CAD build for the part. Positions are in the model's coordinates, mm. Face numbers are marked on the shaded views. Coordinates: 2 decimals unless noted, no trailing zeros. Order: outer loops, then holes, each group sorted by start corner. A loop starts at its lowest first (then second) coordinate and runs counter-clockwise, first axis right, second up. Notation, with made-up numbers: (75, 3.25) -> (115, 3.25) arc R8 ccw to (115, 10.25) -> close; hole circle Ø4 at (81.25, 45.5). An arc over 180 degrees is marked (long way). Use one line per item in the form item = value. Start each with the question number.
from build123d import *

# Parameters (mm, degrees)
F1_DEPTH = 60
F2_R     = 26.678258
F3_DEPTH = 25


with BuildPart() as f1:
    # F0 (on Front) → F1 (new body)
    with BuildSketch(Plane.XZ):
        with BuildLine():
            Line((4.061145, 78.143452), (-15.64565, 78.143452))
            ThreePointArc((-15.64565, 78.143452), (-26.968879, 75.432115), (-35.83602, 67.886212))
            Line((-35.83602, 67.886212), (-50.667426, 47.57444))
            ThreePointArc((-50.667426, 47.57444), (-54.244252, 40.585414), (-55.477056, 32.831681))
            Line((-55.477056, 32.831681), (-55.477056, 3.143452))
            ThreePointArc((-55.477056, 3.143452), (-48.154725, -14.534217), (-30.477056, -21.856548))
            Line((-30.477056, -21.856548), (19.522944, -21.856548))
            ThreePointArc((19.522944, -21.856548), (37.200614, -14.534217), (44.522944, 3.143452))
            Line((44.522944, 3.143452), (44.522944, 32.623266))
            ThreePointArc((44.522944, 32.623266), (43.231192, 40.555414), (39.489426, 47.667853))
            Line((39.489426, 47.667853), (24.027628, 68.188039))
            ThreePointArc((24.027628, 68.188039), (15.216533, 75.516591), (4.061145, 78.143452))
        make_face()
    extrude(amount=F1_DEPTH)

    # F2 (on face) → F3 (cut)
    with BuildSketch(Plane(origin=(0, 0, 0), x_dir=(-1, 0, 0), z_dir=(0, 1, 0))):
        with Locations((6.659664, 24.698926)):
            Circle(F2_R)
    extrude(amount=-F3_DEPTH, mode=Mode.SUBTRACT)


solid = f1.part
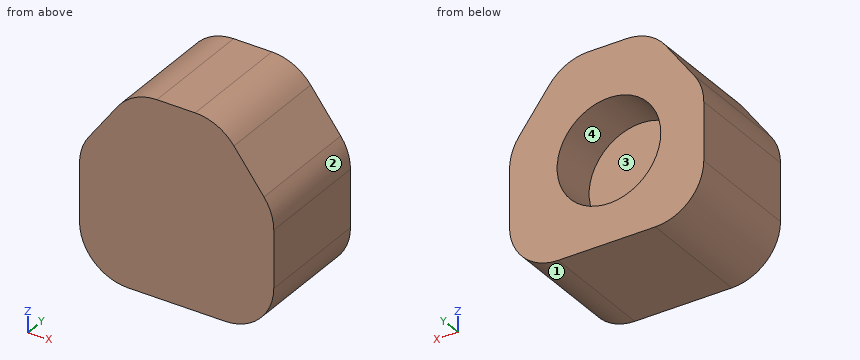
1) Cut at A-A on y = -6. Give the cut face in (x, z).
2) Cut at C-C on y = -40.5. Give the cut face in (x, z), then the cut area to 3 significant figures.
3) Cut at B-B on x = 1. Give the cut face in (y, z), then the cut area to 3 significant figures.
4) Two-plate mould, pull along Z, no slides. Class the marked faces 1, 2, 3 and 4: released by +Z, released by -Z, zero draft, split by the parting line, or undercut.
5) Probe L1, parallel to Y at x = -13, z = 45; L2, parallel to Z at x = -13, y = -13; L3, parallel to Z at x = -21.5, y = -10. List the from-to ranges inside material, lowest first.
6) Drop flat-ended pins along their axis: P1, Ø5, axis at x = 7, z = 10, coming from the +Y side; P2, Ø10, axis at y = -52, z = 50, coming from the -X side; P3, Ø12, axis at y = -46, z = 66, coming from the +X side. Give the stop position or say it passes through.
7) Cut at D-D on z = 45.5. Give the cut face in (x, y).
Values follow:
q1.outline = (-55.48, 3.14) arc R25 ccw to (-30.48, -21.86) -> (19.52, -21.86) arc R25 ccw to (44.52, 3.14) -> (44.52, 32.62) arc R25 ccw to (39.49, 47.67) -> (24.03, 68.19) arc R25 ccw to (4.06, 78.14) -> (-15.65, 78.14) arc R25 ccw to (-35.84, 67.89) -> (-50.67, 47.57) arc R25 ccw to (-55.48, 32.83) -> close; hole circle Ø53.36 at (-6.66, 24.7)
q2.outline = (-55.48, 3.14) arc R25 ccw to (-30.48, -21.86) -> (19.52, -21.86) arc R25 ccw to (44.52, 3.14) -> (44.52, 32.62) arc R25 ccw to (39.49, 47.67) -> (24.03, 68.19) arc R25 ccw to (4.06, 78.14) -> (-15.65, 78.14) arc R25 ccw to (-35.84, 67.89) -> (-50.67, 47.57) arc R25 ccw to (-55.48, 32.83) -> close
q2.area = 8,650 mm^2
q3.outline = (-60, -21.86) -> (0, -21.86) -> (0, -0.86) -> (-25, -0.86) -> (-25, 50.25) -> (0, 50.25) -> (0, 78.14) -> (-60, 78.14) -> close
q3.area = 4,720 mm^2
q4.face_1 = released by -Z
q4.face_2 = released by +Z
q4.face_3 = undercut
q4.face_4 = undercut
q5.L1 = -60 to -25
q5.L2 = -21.86 to -1.21, 50.61 to 78.14
q5.L3 = -21.86 to 2.53, 46.87 to 77.45
q6.P1 = -25
q6.P2 = -52.32
q6.P3 = 30.2
q7.outline = (-52.03, -60) -> (40.95, -60) -> (40.95, 0) -> (10.04, 0) -> (10.04, -25) -> (-23.36, -25) -> (-23.36, 0) -> (-52.03, 0) -> close
